Can you work these out from the model? Positions are in its coordinate system, mm. Face numbers are marked on the shaded views. A direction names the side the tool comes from. Give positions to 0.01 mm unless a question says otherwise; leave off trailing zeros. Order: outer loops, then holes, each group sorted by start corner. A loop starts at its lowest first (then second) coordinate and runs counter-clockwise, first axis right, second up. Notation, with made-up numbers: M 79,7 L 118,7 A27 cw 118,31 Z; hole C -27.75,41.5 d11. An arc over 180 degrees is marked long. Answer as a JSON object with one key per item and string values.
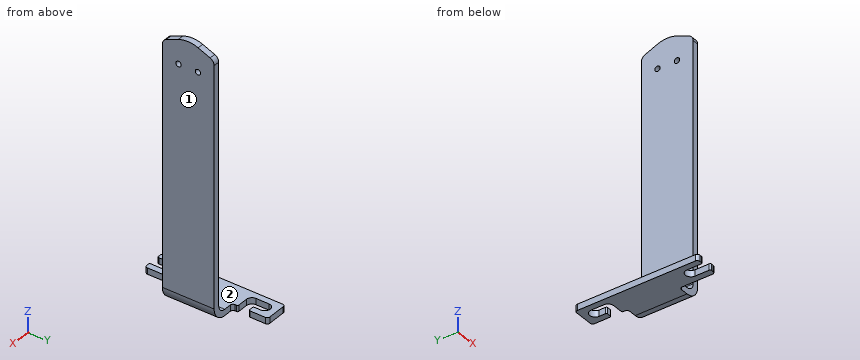
Autodesk Inventor part; units mm, degrees
ref_plane "YZ Plane" through (0, 0, 0) normal (1, 0, 0) x (0, 1, 0)
ref_plane "XZ Plane" through (0, 0, 0) normal (0, 1, 0) x (-1, 0, 0)
ref_plane "XY Plane" through (0, 0, 0) normal (0, 0, 1) x (1, 0, 0)
sketch "Sketch3" plane through (0, 0, 0) normal (0, 0, 1) x (1, 0, 0)
  line L0 (9, -47.5) -> (-9, -47.5)
  line L1 (-9, -47.5) -> (-9, 47.5)
  line L2 (-9, 47.5) -> (9, 47.5)
  line L3 (9, 47.5) -> (9, -47.5)
  line L4 (9, -47.5) -> (-9, 47.5) construction
  line L5 (-9, -47.5) -> (9, 47.5) construction
  line L6 (9, 47.5) -> (14, 47.5)
  line L7 (14, 47.5) -> (14, -47.5)
  line L8 (14, -47.5) -> (9, -47.5)
  line L9 (9, -47.5) -> (9, 47.5)
  point P0 (0, 0)
  dimension "d10" = 18
  dimension "d11" = 95
  dimension "d25" = 5
extrude "Plate2" add sketch "Sketch3" along normal blind 4.7625 contours L0 L1 L2 L3
sketch "Sketch4" plane through (0, 0, 4.7625) normal (0, 0, 1) x (1, 0, 0)
  line L0 (-9, -47.5) -> (-9, 47.5) construction
  line L1 (0, 28.5) -> (0, 38.5) construction
  line L2 (4.2, 28.5) -> (4.2, 38.5)
  line L3 (-4.2, 38.5) -> (-4.2, 28.5)
  arc A0 (-4.2, 28.5) -> (4.2, 28.5) centre (0, 28.5) ccw
  arc A1 (4.2, 38.5) -> (-4.2, 38.5) centre (0, 38.5) ccw
  line L4 (0, -35.5) -> (0, -47.5) construction
  line L5 (-9, -47.5) -> (9, -47.5)
  line L6 (-4.2, -35.5) -> (-4.2, -47.5)
  line L7 (4.2, -47.5) -> (4.2, -35.5)
  arc A2 (4.2, -35.5) -> (-4.2, -35.5) centre (0, -35.5) ccw
  arc A3 (-4.2, -47.5) -> (4.2, -47.5) centre (0, -47.5) ccw
  line L8 (0, -41) -> (0, -35.5) construction
  line L9 (0, 28.5) -> (9, 28.5) construction
  line L10 (0, 32.7) -> (9, 32.7)
  line L11 (9, 24.3) -> (0, 24.3)
  arc A4 (0, 32.7) -> (0, 24.3) centre (0, 28.5) ccw
  arc A5 (9, 24.3) -> (9, 32.7) centre (9, 28.5) ccw
  line L12 (9, 47.5) -> (9, -47.5)
  line L13 (-9, 47.5) -> (9, 47.5)
  point P0 (0, 0)
  point P1 (0, 33.5)
  point P2 (0, -41.5)
  point P3 (4.5, 28.5)
  point P4 (0, 42.7)
  point P5 (4.2, 32.7)
  point P6 (0, 24.3)
  dimension "d15" = 10
  dimension "d61" = 4.2
  dimension "d62" = 12
  dimension "d63" = 4.8
  dimension "d64" = 4.8
extrude "Extrusion2" cut sketch "Sketch4" against normal through all contours A0 A4 L10 L2 | L2 L10 L12 L11 A0 | L10 A4 L3 A1 L2 | L6 A2 L7 L5
fillet "Fillet3" radius 1 5 edges at (-4.2, -47.5, 2.3813) (4.2, -47.5, 2.3813) (9, 32.7, 2.3813) (9, 24.3, 2.3813) (4.2, 32.7, 2.3813)
fillet "Fillet4" radius 2 4 edges at (-9, 47.5, 2.3813) (-9, -47.5, 2.3813) (9, 47.5, 2.3813) (9, -47.5, 2.3813)
sketch "Sketch5" plane through (0, 0, 4.7625) normal (0, 0, 1) x (1, 0, 0)
  line L0 (16.8875, -20) -> (9, -20)
  line L1 (9, -20) -> (9, 20)
  line L2 (9, 20) -> (16.8875, 20)
  line L3 (16.8875, 20) -> (16.8875, -20)
  line L4 (16.8875, -20) -> (9, 20) construction
  line L5 (9, -20) -> (16.8875, 20) construction
  line L6 (28, 20.7219) -> (28, -16.4847) construction
  line L7 (9, 24.3) -> (9, -47.5)
  point P0 (0, 0)
  point P1 (12.9438, 0)
  point P2 (14, -29.8149)
  dimension "d20" = 40
  dimension "d21" = 28
  dimension "d22" = 11.1125
extrude "Extrusion3" add sketch "Sketch5" against normal up to surface (4.7625 mm away)
sketch "Sketch6" plane through (23.2375, 20, 11.1125) normal (1, 0, 0) x (0, 1, 0)
  line L0 (-40, 0) -> (0, 0)
  line L1 (0, 0) -> (0, 173.65)
  line L2 (0, 173.65) -> (-40, 173.65)
  line L3 (-40, 173.65) -> (-40, 0)
edge flange "Flange1" height 180 angle 90 thickness 4.7625 bend radius 6.35 thickness toward (1, 0, 0) relief tear relief width 4.7625 relief depth 2.3813 edges at (16.8875, 0, 4.7625) wall of the first edge with corners at (23.2375, -20, 11.1125) (23.2375, 20, 11.1125) (23.2375, 20, 184.7625) (23.2375, -20, 184.7625)
bend "Bend1"
corner "Corner1"
sketch "Sketch7" plane through (23.2375, -20, 184.7625) normal (-1, 0, 0) x (0, 0, 1)
  line L0 (-173.65, 40) -> (-173.65, 0) construction
  line L1 (0, 0) -> (-173.65, 0) construction
  line L2 (0, 0) -> (0, 40)
  line L3 (0, 40) -> (-173.65, 40) construction
  line L4 (0, 40) -> (13.3636, 40)
  line L5 (13.3636, 40) -> (18.4776, 27.6537)
  line L6 (18.4776, 12.3463) -> (13.3636, 0)
  line L7 (13.3636, 0) -> (0, 0)
  line L8 (0, 0) -> (0, 40) construction
  circle A0 centre (0, 20) radius 17 construction
  arc A1 (18.4776, 12.3463) -> (18.4776, 27.6537) centre (0, 20) ccw
  line L9 (0, 27.5) -> (0, 12.5) construction
  line L10 (0, 0) -> (0, 40) construction
  circle A2 centre (0, 27.5) radius 5 construction
  circle A3 centre (0, 12.5) radius 5 construction
  circle A4 centre (0, 20) radius 15 construction
  point P0 (-184.7625, 20)
  point P1 (21.6478, 20)
  dimension "d36" = 135
  dimension "d44" = 3
  dimension "d45" = 3
  dimension "d49" = 15
  dimension "d50" = 10
  dimension "d51" = 10
  dimension "d59" = 30
extrude "Extrusion4" add sketch "Sketch7" against normal up to surface (4.7625 mm away)
fillet "Fillet7" radius 5 2 edges at (25.6188, 20, 198.1261) (25.6188, -20, 198.1261)
fillet "Fillet8" radius 2 2 edges at (9, 20, 2.3813) (9, -20, 2.3813)
hole "Hole1" at (23.2375, 7.5, 184.7625) at (23.2375, -7.5, 184.7625) direction (1, 0, 0) diameter 4.134 end through all
equation "\"d45\" = d44"
equation "\"d57\" = Thickness"
equation "\"d7\" = Thickness"
equation "\"d26\" = BendReliefWidth"
equation "\"d27\" = BendReliefDepth"
equation "\"d28\" = MinimumRemnant"
equation "\"d29\" = TransitionRadius"
equation "\"d32\" = BendRadius"
equation "\"d33\" = CornerReliefSize"
equation "\"d34\" = GapSize"
equation "\"d35\" = JacobiRadiusSize"
equation "\"BendReliefWidth\" = Thickness"
equation "\"BendReliefDepth\" = 0.5 * Thickness"
equation "\"CornerReliefSize\" = 4 * Thickness"
equation "\"MinimumRemnant\" = 2 * Thickness"
equation "\"TransitionRadius\" = BendRadius"
equation "\"JacobiRadiusSize\" = BendRadius"
equation "\"GapSize\" = Thickness"
properties part number "Spool Holder Left" material "Aluminum 6061"
1) I need wall thicknesses on L1, parallel to X at y = 2.5, z = 36; L2, parallel to Z at x = 26, y = -7; L3, parallel to Z at x = -6, y = -40.5. Which ranges of each line are inside material? Lowest first, please.
Results found:
{"L1": "x = 23.24 to 28", "L2": "z = 4.75 to 182.76, 186.77 to 203.5", "L3": "z = 0 to 4.76"}
2) I'm going to push flat-ended pins straight in: pin 1 Ø10 at (x, z) = (19, 72) entering from +Y; pin 2 Ø1.4 at (y, z) = (38.5, 2) entering from +X; pin 3 Ø5.5 at (y, z) = (-7.5, 184.76) entering from -X. Where does each tip first touch, or does it pass through?
Results found:
{"pin 1": "stops at y = 20", "pin 2": "stops at x = 9", "pin 3": "stops at x = 23.24"}
3) I want a section at B-B on z = 106. Write out the boundary of the cut face in (x, y).
Results found:
{"outline": "M 23.24,-20 L 28,-20 L 28,20 L 23.24,20 Z"}
4) For the marked faces 1 and 2, which set-ups out of +Z, -Z, +X, -X, +Y, -Y let a thin tool reach every point of the face, with its end or its side?
Results found:
{"face 1": "+Z, -Z, +X, +Y, -Y", "face 2": "+Z, -X, +Y, -Y"}
